```python
from build123d import *

# Parameters (mm, degrees)
SKETCH1_R            = 5
SHAFT_DEPTH          = 177.8
SKETCH2_W            = 15.875
SKETCH2_H            = 3.175
SHAFT_KEY_MALE_DEPTH = 7.62
SKETCH3_R            = 1.5875
BOLT_BORE_DEPTH      = 50.8
SKETCH4_R            = 4
CUT_EXTRUDE1_DEPTH   = 25.4


with BuildPart() as part:
    # Sketch1 → Shaft (new body)
    with BuildSketch(Plane(origin=(0, 0, 0), x_dir=(0, 0, -1), z_dir=(1, 0, 0))):
        Circle(SKETCH1_R)
    extrude(amount=SHAFT_DEPTH)

    # Sketch2 → Shaft Key Male (add)
    with BuildSketch(Plane(origin=(177.8, 0, 0), x_dir=(0, 0, -1), z_dir=(1, 0, 0))):
        Rectangle(SKETCH2_W, SKETCH2_H)
    extrude(amount=-SHAFT_KEY_MALE_DEPTH)

    # Sketch3 → Bolt Bore (cut)
    with BuildSketch(Plane(origin=(177.8, 0, 0), x_dir=(0, 0, -1), z_dir=(1, 0, 0))):
        Circle(SKETCH3_R)
    extrude(amount=-BOLT_BORE_DEPTH, mode=Mode.SUBTRACT)

    # Sketch4 → Cut-Extrude1 (cut)
    with BuildSketch(Plane.ZY):
        Circle(SKETCH4_R)
    extrude(amount=-CUT_EXTRUDE1_DEPTH, mode=Mode.SUBTRACT)

    # Sketch5 → Revolve1 (revolve)
    with BuildSketch(Plane(origin=(0, 0, 0), x_dir=(1, 0, 0), z_dir=(0, 1, 0)), mode=Mode.PRIVATE) as revolve1_sk:
        Polygon((144.055202203, 0), (15.578475915, 0), (15.578475915, -7.096721058), (39.957910275, -7.096721058), (39.957910275, -9.367671796), (104.670198298, -9.367671796), (104.670198298, -7.475212847), (124.236525445, -7.475212847), (124.236525445, -5), (144.055202203, -5), align=None)
    revolve(revolve1_sk.sketch.rotate(Axis((144.055202203, 0, 0), (-1, 0, 0)), 180), axis=Axis((144.055202203, 0, 0), (-1, 0, 0)))


solid = part.part
```
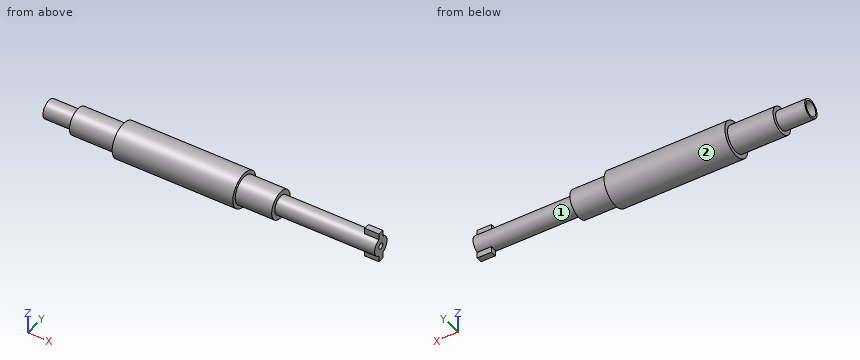
Source: CAD feature listing. Evaluate the final solid. Frame: model axes, mm. Face numbers are marked on the shaded views. Give positions to 0.01 mm unless a question says otherwise; leave off trailing zeros. Write each loop counter-clockwise with the first axis right and the second up, starting at its lowest first coordinate (ties: lowest second). Pieces come first, ordered by that corner, then holes. Notation, with made-up numbers: (65, 84.25) - (107, 84.25) arc R8 cw to (107, 95.25) - close; hole circle Ø9 at (43, 30). An arc over 180 degrees is marked (long way). One line per item, written item: value. Start each with the question number.
Q1. Draft query along X for the marked faces 1 and 2. Return one class per face: +X half, -X half, draft (parallel to the pull), parting line (faces both ways), or undercut.
Q2. Section query B-B, the plane z = 0. Return the cut outline in (x, y).
Q3. Material intervals for probe 1 along Y at (x, z) = (8, 0); probe 2 along X at (y, z) = (-2, -5.25); probe 3 along X at (y, z) = (6.5, 6.5), sorted ascending. Write a range as from..to.
Q4. Section query D-D, the plane x = 51.5. Return the cut outline in (y, z).
Q5. Section query C-C, the plane x = 118.5. Return the cut outline in (y, z), then the cut area to 3 significant figures.
Q6. First-contact query: pin 1 Ø1.6 at (x, y) = (174.5, 0) entering from -Z; pin 2 Ø3.5 at (x, y) = (174.5, 0) entering from +Z; pin 3 Ø3.5 at (x, z) = (175.5, -7) entering from +Y. Flat tips, straight axial feed; report the tip coordinate or a pass-through.
Answer:
1. face 1: undercut
1. face 2: draft
2. outline: (0, -5) - (15.58, -5) - (15.58, -7.1) - (39.96, -7.1) - (39.96, -9.37) - (104.67, -9.37) - (104.67, -7.48) - (124.24, -7.48) - (124.24, -5) - (177.8, -5) - (177.8, -1.59) - (144.06, -1.59) - (144.06, 1.59) - (177.8, 1.59) - (177.8, 5) - (124.24, 5) - (124.24, 7.48) - (104.67, 7.48) - (104.67, 9.37) - (39.96, 9.37) - (39.96, 7.1) - (15.58, 7.1) - (15.58, 5) - (0, 5) - (0, 4) - (15.58, 4) - (15.58, -4) - (0, -4) - close
3. probe 1: y = -5..-4, 4..5
3. probe 2: x = 15.58..124.24
3. probe 3: x = 39.96..104.67
4. outline: circle Ø18.74 at (0, 0)
5. outline: circle Ø14.95 at (0, 0)
5. area: 176 mm2
6. pin 1: stops at z = -7.94
6. pin 2: stops at z = 7.94
6. pin 3: stops at y = 1.59
